Model file for the job. Use its own axes, mm. Face numbers are marked on the shaded views. A direction names the side the tool comes from. Coordinates: 2 decimals unless noted, no trailing zeros. Order: outer loops, then holes, each group sorted by start corner. A loop starts at its lowest first (then second) coordinate and runs counter-clockwise, first axis right, second up. Notation, with made-up numbers: (65.25, 39.5) -> (97.25, 39.5) arc R22 cw to (97.25, 74.5) -> close; hole circle Ø2 at (15, -2). An arc over 180 degrees is marked (long way). Use CSV: the item, a comma, the result in double quotes. Start each with the question number.
(1) Cut at A-A on y = -3.25. Write the cut outline in (x, z).
(2) Pin check, flat tips, straight feed: pin 1 Ø1.5 at (y, z) = (2.5, 15.5) entering from -X; pin 2 Ø1.5 at (x, z) = (0.5, 6) entering from +Y (3 decimals). Stop position of each tip, or through.
(3) Cut at D-D on z = 4.75. Write the cut outline in (x, y) (3 decimals).
(4) Cut at B-B on y = 0. Write the cut outline in (x, z) (3 decimals), plus the area to 3 significant figures.
(5) Probe L1, parallel to Z at x = -0.75, y = 2.75; L2, parallel to Y at x = -1.5, z = 6; L3, parallel to Y at x = 1.75, z = 7.75. List the from-to ranges inside material, lowest first.
(6) Tool access for the marked faces 1 and 2: list every direction of +Z, -Z, +X, -X, +Y, -Y with a clear straight run to the whole face (end or side of a thin tool).
(7) Pull direction Z, two halves, no side cores. Call the marked faces 3, 4, 5 and 6: pulls with the +Z half, pulls with the -Z half, needs draft (parallel to the pull), parting line crosses it, or undercut.
```python
from build123d import *

# Parameters (mm, degrees)
SKETCH1_R           = 1.905
BOSS_EXTRUDE1_DEPTH = 15.24
SKETCH3_R           = 3.81
BOSS_EXTRUDE2_DEPTH = 2.54


with BuildPart() as part:
    # Sketch1 → Boss-Extrude1 (new body)
    with BuildSketch(Plane.XY):
        Circle(SKETCH1_R)
    extrude(amount=BOSS_EXTRUDE1_DEPTH)

    # Sketch3 → Boss-Extrude2 (add)
    with BuildSketch(Plane.XY.offset(15.24)):
        Circle(SKETCH3_R)
    boss_extrude2 = extrude(amount=BOSS_EXTRUDE2_DEPTH)

    # Mirror1: Boss-Extrude2 across plane
    add(boss_extrude2.mirror(Plane.XY.offset(7.62)))


solid = part.part
```
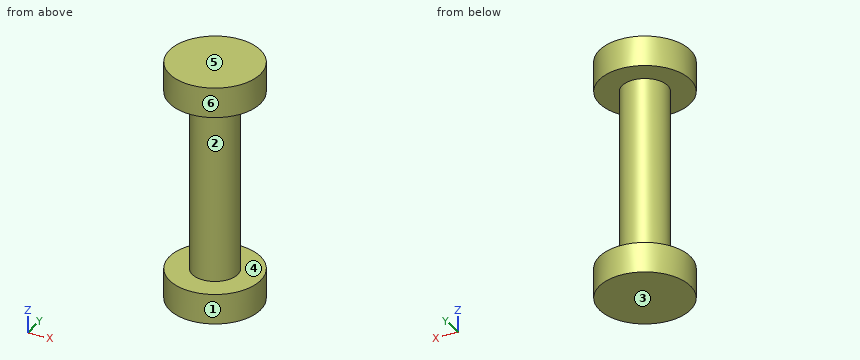
Outcome:
1,outline,"(-1.99, -2.54) -> (1.99, -2.54) -> (1.99, 0) -> (-1.99, 0) -> close; (-1.99, 15.24) -> (1.99, 15.24) -> (1.99, 17.78) -> (-1.99, 17.78) -> close"
2,pin 1,"x = -3.38"
2,pin 2,"y = 1.905"
3,outline,"circle Ø3.81 at (0, 0)"
4,outline,"(-3.81, -2.54) -> (3.81, -2.54) -> (3.81, 0) -> (1.905, 0) -> (1.905, 15.24) -> (3.81, 15.24) -> (3.81, 17.78) -> (-3.81, 17.78) -> (-3.81, 15.24) -> (-1.905, 15.24) -> (-1.905, 0) -> (-3.81, 0) -> close"
4,area,"96.8 mm2"
5,L1,"-2.54 to 0, 15.24 to 17.78"
5,L2,"-1.17 to 1.17"
5,L3,"-0.75 to 0.75"
6,face 1,"+Z, -Z"
6,face 2,"none"
7,face 3,"pulls with the -Z half"
7,face 4,"undercut"
7,face 5,"pulls with the +Z half"
7,face 6,"needs draft"
